Source: CAD feature listing. Evaluate the final solid. Frame: model axes, mm. A direction names the side the tool comes from. Coordinates: 2 decimals unless noted, no trailing zeros. Loops run counter-clockwise (first coordinate to the right, second up) from the corner with the lowest first, then second, coordinate; pieces in that order, holes last.
Item 1: Section query A-A, the plane z = 2. Return the cut outline in (x, y), then the cut area to 3 significant figures.
Item 2: Section query B-B, the plane x = -10. Return the cut outline in (y, z).
Item 3: Reachability of faces 1 (the flat face through (-2, 6, 18)), 2 (the flat face through (4, 10, -3)), 3 (the flat face through (-6.3, 10.4, 1.5)), 4 (the cylindrical face through (0.69, -3.1, -10.14)), 5 (the cylindrical face through (-6, 0, 9)) from +Z, -Z, +X, -X, +Y, -Y: full face, straight path, thin tool, end or side. Return the list, or none.
Item 4: Line query: probe 1 along Y at (x, z) = (0, -9.25) (3 decimals); probe 2 along Z at (x, y) = (8, -5.5); probe 3 along Z at (x, y) = (2.5, -15.5). Output: solid intervals per line, ascending.
Item 5: Section query D-D, the plane z = -9. Return the cut outline in (x, y) (3 decimals).
Item 6: Pin query (flat end, axial travel): pin 1 Ø10 at (x, y) = (8.5, -10.5) entering from +Z; pin 2 Ø6 at (x, z) = (-7.5, 11.5) entering from -Y; pin 3 Ø11 at (x, y) = (0, 0) entering from -Z; pin 4 Ø8 at (x, y) = (8.5, 13.5) entering from -Z. Return the tip coordinate at first contact, or that it passes through.
Item 7: Section query C-C, the plane y = -12.5. Return the cut outline in (x, z), then the cut area to 3 significant figures.
Item 8: Pull-direction query (Z, two-part tool) for faces 6 (the cylindrical face through (12.932, -5.362, 0.74)), 7 (the cylindrical face through (-7.493, 0.33, 6.986)), 8 (the flat face through (-8, -12, 0)); classes: +Z half, -Z half, draft (parallel to the pull), parting line (faces both ways), or undercut.
```python
from build123d import *

# Parameters (mm, degrees)
F1_DEPTH  = 6
F2_R      = 14
F2_R_2    = 12
F3_DEPTH  = 1.5
F4_R      = 10.5
F5_DEPTH  = 3
F7_R      = 11
F8_DEPTH  = 17
F10_R     = 7.5
F11_DEPTH = 2
F13_R     = 8
F14_DEPTH = 10
F17_D     = 6.35
F18_R     = 6
F19_DEPTH = 18


with BuildPart() as f1:
    # F0 (on Top) → F1 (new body)
    with BuildSketch(Plane.XY):
        with BuildLine():
            Line((15, -9.949874), (15, 9.949874))
            ThreePointArc((15, 9.949874), (0, 18), (-15, 9.949874))
            Line((-15, 9.949874), (-15, -9.949874))
            ThreePointArc((-15, -9.949874), (0, -18), (15, -9.949874))
        make_face()
    extrude(amount=F1_DEPTH)

    # F2 (on Top) → F3 (cut)
    with BuildSketch(Plane.XY):
        Circle(F2_R)
        Circle(F2_R_2, mode=Mode.SUBTRACT)
    extrude(amount=F3_DEPTH, mode=Mode.SUBTRACT)

    # F4 (on Top) → F5 (join)
    with BuildSketch(Plane.XY):
        Circle(F4_R)
    extrude(amount=-F5_DEPTH)

    # F7 (on offset) → F8 (join)
    with BuildSketch(Plane(origin=(0, 0, -3), x_dir=(1, 0, 0), z_dir=(0, 0, -1))):
        Circle(F7_R)
    extrude(amount=F8_DEPTH)

    # F10 (on offset) → F11 (join)
    with BuildSketch(Plane.XY.offset(6)):
        Circle(F10_R)
    extrude(amount=F11_DEPTH)

    # F13 (on offset) → F14 (join)
    with BuildSketch(Plane.XY.offset(8)):
        Circle(F13_R)
    extrude(amount=F14_DEPTH)

    # F17 (through all)
    with Locations(Plane.XY.offset(18)):
        with Locations((0, 0)):
            Hole(F17_D / 2)

    # F18 (on offset) → F19 (cut)
    with BuildSketch(Plane.XY.offset(18)):
        Circle(F18_R)
    extrude(amount=-F19_DEPTH, mode=Mode.SUBTRACT)


solid = f1.part
```
Verdict:
1. outline: (-15, -9.95) arc R18 ccw to (15, -9.95) - (15, 9.95) arc R18 ccw to (-15, 9.95) - close; hole circle Ø12 at (0, 0)
1. area: 824 mm2
2. outline: (-14.97, 0) - (-9.8, 0) - (-9.8, 1.5) - (-6.63, 1.5) - (-6.63, 0) - (-3.2, 0) - (-3.2, -3) - (-4.58, -3) - (-4.58, -20) - (4.58, -20) - (4.58, -3) - (3.2, -3) - (3.2, 0) - (6.63, 0) - (6.63, 1.5) - (9.8, 1.5) - (9.8, 0) - (14.97, 0) - (14.97, 6) - (-14.97, 6) - close
3. face 1: +Z, +X, -X, +Y, -Y
3. face 2: none
3. face 3: -Z
3. face 4: +Z, -Z
3. face 5: +Z
4. probe 1: y = -11 to -3.175, 3.175 to 11
4. probe 2: z = -20 to 6
4. probe 3: z = 0 to 6
5. outline: circle Ø22 at (0, 0); hole circle Ø6.35 at (0, 0)
6. pin 1: stops at z = 6
6. pin 2: stops at y = -6.61
6. pin 3: stops at z = -20
6. pin 4: stops at z = 0
7. outline: (-12.95, 0) - (-6.3, 0) - (-6.3, 1.5) - (6.3, 1.5) - (6.3, 0) - (12.95, 0) - (12.95, 6) - (-12.95, 6) - close
7. area: 137 mm2
8. face 6: draft
8. face 7: undercut
8. face 8: -Z half
